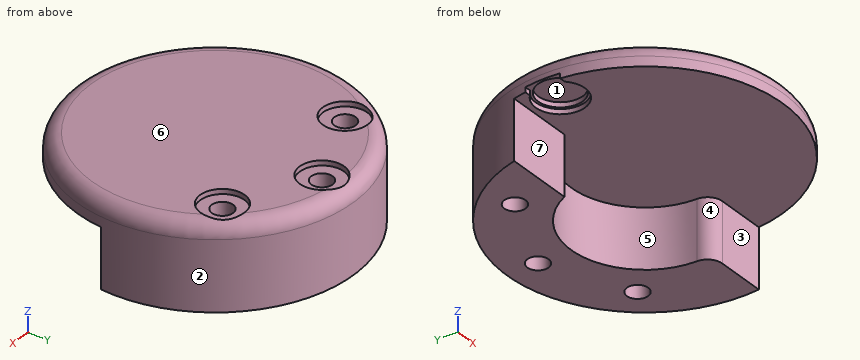
from build123d import *

# Parameters (mm, degrees)
SKETCH_1_R           = 28
EXTRUDE_1_DEPTH      = 15
CUT_EXTRUDE_START    = -22
CUT_EXTRUDE_1_DEPTH  = 22
EXTRUDE_2_DEPTH      = 2
EXTRUDE_2_DEPTH_BACK = 3
SKETCH_3_R           = 28
CUT_EXTRUDE_2_DEPTH  = 1
SKETCH_5_R           = 4.5
CUT_EXTRUDE_3_DEPTH  = 1
SKETCH_7_R           = 2.15
CUT_EXTRUDE_4_DEPTH  = 18
SKETCH_9_R           = 4.5
CUT_EXTRUDE_6_DEPTH  = 1
FILLET_5_R           = 3


with BuildPart() as part:
    # 草图1 → 凸台-拉伸1 (new body)
    with BuildSketch(Plane.XY):
        Circle(SKETCH_1_R)
    extrude(amount=EXTRUDE_1_DEPTH)

    # 草图2 → 切除-拉伸1 (cut)
    with BuildSketch(Plane.XY.offset(15).offset(CUT_EXTRUDE_START)):
        with BuildLine():
            Line((14.996539752, -0.000319471), (14.996539752, -2.262315411))
            Line((14.996539752, -2.262315411), (27.908456227, -2.262315411))
            ThreePointArc((27.908456227, -2.262315411), (-4.220435571, -27.680099776), (-27.314529778, 6.157634529))
            Line((-27.314529778, 6.157634529), (-13.674053592, 6.157634529))
            ThreePointArc((-13.674053592, 6.157634529), (3.149181128, 14.66215751), (14.996539752, -0.000319471))
        make_face()
    extrude(amount=CUT_EXTRUDE_1_DEPTH, mode=Mode.SUBTRACT)

    # 草图3 → 凸台-拉伸2 (add, two sides: drawn at the far end of the back side and taken through both)
    with BuildSketch(Plane.XY.offset(15).offset(-EXTRUDE_2_DEPTH_BACK)):
        with Locations(Location((0, 0, 0), (0, 0, 167.295928936))):
            Circle(SKETCH_3_R)
    extrude(amount=EXTRUDE_2_DEPTH + EXTRUDE_2_DEPTH_BACK)

    # 草图4 → 切除-拉伸2 (cut)
    with BuildSketch(Plane(origin=(0, 0, 12), x_dir=(-1, 0, 0), z_dir=(0, 0, -1))):
        with BuildLine():
            Line((26.535533906, 3.535533906), (27.775888825, 3.535533906))
            ThreePointArc((27.775888825, 3.535533906), (28, 0), (27.775888825, -3.535533906))
            Line((27.775888825, -3.535533906), (26.535533906, -3.535533906))
            ThreePointArc((26.535533906, -3.535533906), (18, 0), (26.535533906, 3.535533906))
        make_face()
    extrude(amount=-CUT_EXTRUDE_2_DEPTH, mode=Mode.SUBTRACT)

    # 草图5 → 切除-拉伸3 (cut)
    with BuildSketch(Plane(origin=(0, 0, 13), x_dir=(-1, 0, 0), z_dir=(0, 0, -1))):
        with Locations((23, 0)):
            Circle(SKETCH_5_R)
    extrude(amount=-CUT_EXTRUDE_3_DEPTH, mode=Mode.SUBTRACT)

    # 草图7 → 切除-拉伸4 (cut)
    with BuildSketch(Plane.XY):
        with Locations(Location((16.661466638, 13.980630511, 0), (0, 0, 180))):
            Circle(SKETCH_7_R)
        with Locations((-16.661466638, 13.980630511)):
            Circle(SKETCH_7_R)
        with Locations((0, 21.75)):
            Circle(SKETCH_7_R)
    extrude(amount=CUT_EXTRUDE_4_DEPTH, mode=Mode.SUBTRACT)

    # 草图9 → 切除-拉伸6 (cut)
    with BuildSketch(Plane.XY.offset(17)):
        with Locations((0, 21.75)):
            Circle(SKETCH_9_R)
        with Locations((16.661466638, 13.980630511)):
            Circle(SKETCH_9_R)
        with Locations((-16.661466638, 13.980630511)):
            Circle(SKETCH_9_R)
    extrude(amount=-CUT_EXTRUDE_6_DEPTH, mode=Mode.SUBTRACT)

    # 圆角5
    # the kernel refuses this fillet: 3 mm, written as the material it takes off along each edge
    with BuildSketch(Plane(origin=(14.996539752, -2.262315411, -7.462186675), x_dir=(1, 0, 0), z_dir=(0, 0, 1))) as fillet_5_piece_1:
        with BuildLine():
            CenterArc((2.98487467, 3), FILLET_5_R, 182.349232636, 87.650767364)
            Line((-0.012603956, 2.877028929), (-0.312351819, 2.864731822))
            ThreePointArc((-0.312351819, 2.864731822), (-0.3, 2.262002331), (-0.3, 0))
            Line((-0.3, 0), (0, -0.3))
            Line((0, -0.3), (2.98487467, -0.3))
            Line((2.98487467, -0.3), (2.98487467, 0))
        make_face()
    extrude(amount=19.462186675, mode=Mode.SUBTRACT)
    with BuildSketch(Plane(origin=(0, 0, 17), x_dir=(-0.9755189206474555, 0.21991551891311267, 0), z_dir=(0.21991551891311267, 0.9755189206474555, 0))) as fillet_5_piece_2:
        with BuildLine():
            CenterArc((28 - FILLET_5_R, -FILLET_5_R), FILLET_5_R, 0, 90)
            Line((28 - FILLET_5_R, 0), (28, 0))
            Line((28, 0), (28, -FILLET_5_R))
        make_face()
    revolve(axis=Axis((0, 0, 17), (0, 0, 1)), mode=Mode.SUBTRACT)


solid = part.part
Part model, mm, in its own coordinate system. Face numbers are marked on the shaded views. A direction names the side the tool comes from. Coordinates: 2 decimals unless noted, no trailing zeros. Write each loop counter-clockwise with the first axis right and the second up, starting at its lowest first coordinate (ties: lowest second). Pieces come first, ordered by that corner, then holes. Notation, with made-up numbers: M 47,31 L 89,31 A16 cw 89,49 Z; hole C 48.25,89.5 d1. An arc over 180 degrees is marked long. Return JSON: item names as keys, results as strings.
1. Pull direction X, two halves, no side cores. Call the marked faces 1, 2, 3 and 4: pulls with the +X half, pulls with the -X half, needs draft (parallel to the pull), parting line crosses it, or undercut.
Determined:
{"face 1": "undercut", "face 2": "parting line crosses it", "face 3": "needs draft", "face 4": "pulls with the -X half"}
2. Flat gauge pins, fed straight in: pin 1 Ø8 at (x, y) = (0, 21.75) entering from +Z; pin 2 Ø8 at (y, z) = (21.5, 6.5) entering from -X; pin 3 Ø5 at (x, y) = (10, 20) entering from -Z; pin 4 Ø3 at (x, y) = (-23, 0) entering from -Z. Where does each tip first touch, or does it go through?
Determined:
{"pin 1": "z = 16", "pin 2": "x = -21.86", "pin 3": "z = 0", "pin 4": "z = 14"}
3. 3-axis set-ups, long thin cutter, end or side, ignore diameter. For the marked faces 5, 6 and 7: which of +Z, -Z, +X, -X, +Y, -Y reach the whole face in a straight line?
Determined:
{"face 5": "-Z, -Y", "face 6": "+Z, +X, -X, +Y, -Y", "face 7": "-Z, -X, -Y"}
4. Probe L1, parallel to X at y = 13, z = 3.5; L2, parallel to Z at x = -0.5, y = 10; L3, parallel to X at y = 21.75, z = 16.3. List the from-to ranges inside material, lowest first.
Determined:
{"L1": "-24.8 to -18.57, -14.75 to -7.48, 7.48 to 14.75, 18.57 to 24.8", "L2": "12 to 17", "L3": "-15.87 to -4.5, 4.5 to 15.87"}
5. Saw through at A-A, the plane z = 8.75. Write the cut outline in (x, y), then the cut area to 3 significant figures.
Determined:
{"outline": "M -27.31,6.16 L -13.67,6.16 A15 cw 14.98,0.61 A3 ccw 17.98,-2.26 L 27.91,-2.26 A28 ccw Z; hole C -16.66,13.98 d4.3; hole C 0,21.75 d4.3; hole C 16.66,13.98 d4.3", "area": "781 mm²"}
